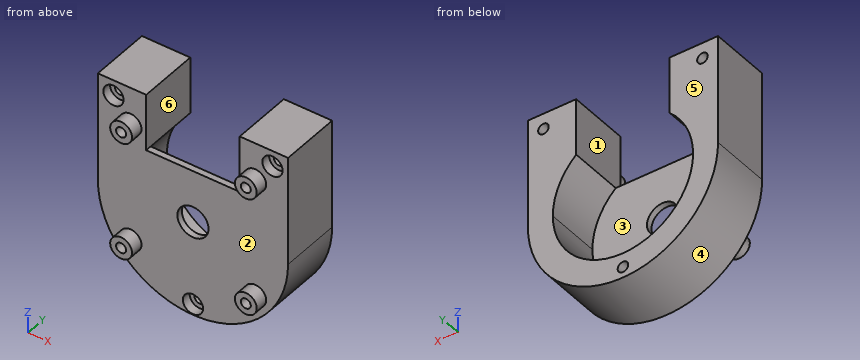
```python
from build123d import *
from build123d.topology import SkipClean

# Parameters (mm, degrees)
BOSS_EXTRUDE1_DEPTH            = 17.5
SKETCH2_R                      = 5
BOSS_EXTRUDE2_DEPTH            = 2
SKETCH3_R                      = 3.5
SKETCH3_R_2                    = 1.6
BOSS_EXTRUDE3_DEPTH            = 4.2
CBORE_FOR_M3_SHCS1_D           = 3.4
CBORE_FOR_M3_SHCS1_DEPTH       = 19.5
CBORE_FOR_M3_SHCS1_CBORE_D     = 6.5
CBORE_FOR_M3_SHCS1_CBORE_DEPTH = 3
CBORE_FOR_M3_SHCS1_TIP         = 1.021463052


with BuildPart() as part:
    # Sketch1 → Boss-Extrude1 (new body)
    with BuildSketch(Plane(origin=(0, 0, 0), x_dir=(1, 0, 0), z_dir=(0, 1, 0))):
        with BuildLine():
            Line((-15, -26.55654345), (-15, -16.770509831))
            ThreePointArc((-15, -16.770509831), (-9.185586535, 20.539595906), (22.5, 0))
            ThreePointArc((22.5, 0), (20.539595906, -9.185586535), (15, -16.770509831))
            Line((15, -16.770509831), (15, -26.55654345))
            ThreePointArc((15, -26.55654345), (26.34150717, -15.374491862), (30.5, 0))
            ThreePointArc((30.5, 0), (0, 30.5), (-30.5, 0))
            ThreePointArc((-30.5, 0), (-26.34150717, -15.374491862), (-15, -26.55654345))
        make_face()
        with BuildLine():
            Line((-15, -35), (-15, -26.55654345))
            ThreePointArc((-15, -26.55654345), (-26.34150717, -15.374491862), (-30.5, 0))
            Line((-30.5, 0), (-30.5, -35))
            Line((-30.5, -35), (-15, -35))
        make_face()
        with BuildLine():
            ThreePointArc((30.5, 0), (26.34150717, -15.374491862), (15, -26.55654345))
            Line((15, -26.55654345), (15, -35))
            Line((15, -35), (30.5, -35))
            Line((30.5, -35), (30.5, 0))
        make_face()
    extrude(amount=-BOSS_EXTRUDE1_DEPTH)

    # Sketch2 → Boss-Extrude2 (add)
    # profile 1 of 2: a face of its own
    with SkipClean():  # the faces are left unmerged after this step: merging them gives an invalid solid
        with BuildSketch(Plane.XZ.offset(17.5)):
            with BuildLine():
                Line((-15, 16.770509831), (15, 16.770509831))
                ThreePointArc((15, 16.770509831), (0, -22.5), (-15, 16.770509831))
            make_face()
            with Locations(Location((0, 0, 0), (0, 0, 270))):
                Circle(SKETCH2_R, mode=Mode.SUBTRACT)
        # profile 2 of 2: a face of its own
        with BuildSketch(Plane.XZ.offset(17.5)):
            with BuildLine():
                Line((30.5, 35), (15, 35))
                Line((15, 35), (15, 16.770509831))
                ThreePointArc((15, 16.770509831), (0, -22.5), (-15, 16.770509831))
                Line((-15, 16.770509831), (-15, 35))
                Line((-15, 35), (-30.5, 35))
                Line((-30.5, 35), (-30.5, 0))
                ThreePointArc((-30.5, 0), (0, -30.5), (30.5, 0))
                Line((30.5, 0), (30.5, 35))
            make_face()
        extrude(amount=BOSS_EXTRUDE2_DEPTH)

    # Sketch3 → Boss-Extrude3 (add)
    # profile 1 of 4: a face of its own
    with SkipClean():  # the faces are left unmerged after this step: merging them gives an invalid solid
        with BuildSketch(Plane.XZ.offset(19.5)):
            with Locations(Location((-20, 23, 0), (0, 0, 270))):
                Circle(SKETCH3_R)
            with Locations(Location((-20, 23, 0), (0, 0, 270))):
                Circle(SKETCH3_R_2, mode=Mode.SUBTRACT)
        # profile 2 of 4: a face of its own
        with BuildSketch(Plane.XZ.offset(19.5)):
            with Locations(Location((20, 23, 0), (0, 0, 270))):
                Circle(SKETCH3_R)
            with Locations(Location((20, 23, 0), (0, 0, 270))):
                Circle(SKETCH3_R_2, mode=Mode.SUBTRACT)
        # profile 3 of 4: a face of its own
        with BuildSketch(Plane.XZ.offset(19.5)):
            with Locations(Location((20, -15, 0), (0, 0, 270))):
                Circle(SKETCH3_R)
            with Locations(Location((20, -15, 0), (0, 0, 270))):
                Circle(SKETCH3_R_2, mode=Mode.SUBTRACT)
        # profile 4 of 4: a face of its own
        with BuildSketch(Plane.XZ.offset(19.5)):
            with Locations(Location((-20, -15, 0), (0, 0, 270))):
                Circle(SKETCH3_R)
            with Locations(Location((-20, -15, 0), (0, 0, 270))):
                Circle(SKETCH3_R_2, mode=Mode.SUBTRACT)
        extrude(amount=BOSS_EXTRUDE3_DEPTH)

    # CBORE for M3 SHCS1
    with Locations(Plane.XZ.offset(19.5)):
        with Locations((0, -27), (25.5, 30), (-25.5, 30)):
            CounterBoreHole(CBORE_FOR_M3_SHCS1_D / 2, CBORE_FOR_M3_SHCS1_CBORE_D / 2, CBORE_FOR_M3_SHCS1_CBORE_DEPTH, depth=CBORE_FOR_M3_SHCS1_DEPTH)
            with Locations((0, 0, -(CBORE_FOR_M3_SHCS1_DEPTH + CBORE_FOR_M3_SHCS1_TIP / 2))):  # 118° drill point
                Cone(0, CBORE_FOR_M3_SHCS1_D / 2, CBORE_FOR_M3_SHCS1_TIP, mode=Mode.SUBTRACT)


solid = part.part
```
Can you work these out from the model? Positions are in its coordinate system, mm. Face numbers are marked on the shaded views. A direction names the side the tool comes from. Give positions to 0.01 mm unless a question says otherwise; leave off trailing zeros. Order: outer loops, then holes, each group sorted by start corner. A loop starts at its lowest first (then second) coordinate and runs counter-clockwise, first axis right, second up. Notation, with made-up numbers: M 4.5,82 L 55.5,82 A28 cw 55.5,118 Z; hole C 60,84.5 d6. An arc over 180 degrees is marked long. Write item = value, one per line. Start each with the question number.
Q1. Will these pins go through, and if not, where does the flat tip stop? pin 1 Ø4.5 at (x, z) = (-25.5, 30) entering from -Y; pin 2 Ø1 at (x, z) = (19.5, 23) entering from -Y; pin 3 Ø6 at (x, y) = (9, -14) entering from -Z; pin 4 Ø3 at (x, z) = (25.5, 30) entering from +Y.
Q2. I need wall thicknesses on probe 1 along X at (y, z) = (-20.3, 23); probe 2 along X at (y, z) = (-18, 0); probe 3 along Z at (x, y) = (0, -17.35). Which ranges of each line are inside material? Lowest first, please. Write a range as [from, to].
Q3. Suppose I cut it at C-C (y = -2.75). Write out the boundary of the cut face in (x, z), plus the area to 3 significant figures.
Q4. We'd pull the mould along X, two halves only. Please class the marked faces 4, 5 and 6: pulls with the +X half, pulls with the -X half, needs draft (parallel to the pull), parting line crosses it, or undercut.
Q5. Suppose I cut it at D-D (z = 23). Write out the boundary of the cut face in (x, y), plus the area to 3 significant figures.
Q6. For the marked faces 1, 2 and 3, which set-ups out of +Z, -Z, +X, -X, +Y, -Y let a thin tool reach every point of the face, with its end or its side?
Q7. Suppose I cut it at A-A (y = -20.75). Write out the boundary of the cut face in (x, z), plus the area to 3 significant figures.
Q8. Suppose I cut it at B-B (z = 30). Write out the boundary of the cut face in (x, y), plus the area to 3 significant figures.
Check result:
q1.pin_1 = -16.5
q1.pin_2 = -19.5
q1.pin_3 = -29.9
q1.pin_4 = through
q2.probe_1 = [-23.5, -21.6], [-18.4, -16.5], [16.5, 18.4], [21.6, 23.5]
q2.probe_2 = [-30.5, -5], [5, 30.5]
q2.probe_3 = [-30.5, -30.25], [-23.75, -22.5]
q3.outline = M -30.5,0 A30.5 ccw 30.5,0 L 30.5,35 L 15,35 L 15,16.77 A22.5 cw long -15,16.77 L -15,35 L -30.5,35 Z; hole C -25.5,30 d3.4; hole C 0,-27 d3.4; hole C 25.5,30 d3.4
q3.area = 1,550 mm2
q4.face_4 = parting line crosses it
q4.face_5 = needs draft
q4.face_6 = undercut
q5.outline = M -30.5,-19.5 L -23.5,-19.5 L -23.5,-23.7 L -21.6,-23.7 L -21.6,-19.5 L -18.4,-19.5 L -18.4,-23.7 L -16.5,-23.7 L -16.5,-19.5 L -15,-19.5 L -15,0 L -30.5,0 Z; M 15,-19.5 L 16.5,-19.5 L 16.5,-23.7 L 18.4,-23.7 L 18.4,-19.5 L 21.6,-19.5 L 21.6,-23.7 L 23.5,-23.7 L 23.5,-19.5 L 30.5,-19.5 L 30.5,0 L 15,0 Z
q5.area = 636 mm2
q6.face_1 = +Z, +Y, -Y
q6.face_2 = -Y
q6.face_3 = +Y
q7.outline = C -20,-15 d7; C -20,23 d7; C 20,-15 d7; C 20,23 d7; hole C -20,-15 d3.2; hole C -20,23 d3.2; hole C 20,-15 d3.2; hole C 20,23 d3.2
q7.area = 122 mm2
q8.outline = M -30.5,-19.5 L -28.75,-19.5 L -28.75,-16.5 L -27.2,-16.5 L -27.2,0 L -30.5,0 Z; M -23.8,-16.5 L -22.25,-16.5 L -22.25,-19.5 L -15,-19.5 L -15,0 L -23.8,0 Z; M 15,-19.5 L 22.25,-19.5 L 22.25,-16.5 L 23.8,-16.5 L 23.8,0 L 15,0 Z; M 27.2,-16.5 L 28.75,-16.5 L 28.75,-19.5 L 30.5,-19.5 L 30.5,0 L 27.2,0 Z
q8.area = 453 mm2
